Work out the finished part from the listing and answer in its coordinate system (mm). Face numbers are marked on the shaded views. A direction names the side the tool comes from. Coordinates: 2 decimals unless noted, no trailing zeros. Order: outer loops, then holes, each group sorted by start corner. A loop starts at its lowest first (then second) coordinate and runs counter-clockwise, first axis right, second up. Notation, with made-up numbers: (63, 68) -> (95, 68) arc R9 cw to (95, 76) -> close; hole circle Ø3 at (-15.5, 88.25). An arc over 180 degrees is marked (long way). Answer as CSV lines item,"result". Start each with the question number.
Item 1: Section A-A (y = 56.5) is taken. Count the separate pieces of the cut face and the enclosed holes in it, then the cut area to 3 significant figures.
Item 2: For a pull along X with two mould halves and no side action, classify the marked faces 1, 2, 3 and 4 as pulls with the +X half, pulls with the -X half, needs draft (parallel to the pull), parting line crosses it, or undercut.
Item 3: Straight lines are drawn through the part: L1, parallel to X at y = 56.75, z = 54; L2, parallel to Z at x = 24, y = 56.75; L3, parallel to Y at x = -36.5, z = 60. For each, find the intervals that lie inside material, in ascending order.
Item 4: Which of the six approach directions +Z, -Z, +X, -X, +Y, -Y give full straight-line access (tool end or side, diameter ignored) to the marked faces 5, 6, 7, 8 and 9?
Item 5: Section D-D (x = 26) is taken. Write down the section's boundary in (y, z).
Item 6: Each of these flat-tipped pins is pushed along its axis until it touches: pin 1 Ø5 at (x, z) = (19, 73) entering from +Y; pin 2 Ø0.7 at (x, y) = (3, 60.5) entering from +Z; pin 3 Ø1.8 at (y, z) = (60, 58) entering from -X. Where does it stop, or does it pass through?
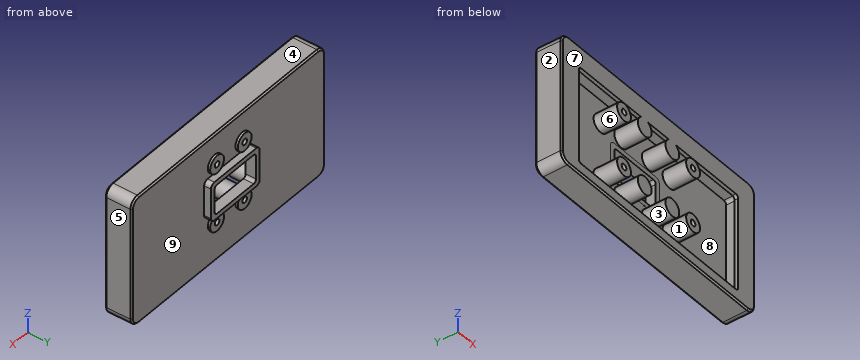
```python
from build123d import *

# Parameters (mm, degrees)
BOSS_EXTRUDE1_START  = 50
BOSS_EXTRUDE1_DEPTH  = 9.2
CHAMFER1_SIZE        = 0.5
CHAMFER2_SIZE        = 0.5
BOSS_EXTRUDE2_START  = 49
BOSS_EXTRUDE2_DEPTH  = 9
BOSS_EXTRUDE3_START  = 50
SKETCH3_R            = 3
BOSS_EXTRUDE3_DEPTH  = 8.01
BOSS_EXTRUDE4_START  = 49
SKETCH4_R            = 1
BOSS_EXTRUDE4_DEPTH  = 9.4
BOSS_EXTRUDE5_START  = 50
SKETCH5_R            = 3
BOSS_EXTRUDE5_DEPTH  = 8.01
BOSS_EXTRUDE6_START  = 49
SKETCH6_R            = 1
BOSS_EXTRUDE6_DEPTH  = 9.4
BOSS_EXTRUDE7_START  = 50
SKETCH7_R            = 3
BOSS_EXTRUDE7_DEPTH  = 8.01
BOSS_EXTRUDE8_START  = 49
SKETCH8_R            = 1
BOSS_EXTRUDE8_DEPTH  = 9.4
BOSS_EXTRUDE9_START  = 50
SKETCH9_R            = 3
BOSS_EXTRUDE9_DEPTH  = 8.01
BOSS_EXTRUDE10_START = 49
SKETCH10_R           = 1
BOSS_EXTRUDE10_DEPTH = 9.4
BOSS_EXTRUDE11_START = 50
SKETCH11_R           = 3
BOSS_EXTRUDE11_DEPTH = 10
BOSS_EXTRUDE12_START = 51.5
SKETCH12_R           = 1
BOSS_EXTRUDE12_DEPTH = 9.5
BOSS_EXTRUDE13_START = 50
SKETCH13_R           = 3
BOSS_EXTRUDE13_DEPTH = 10
BOSS_EXTRUDE14_START = 51.5
SKETCH14_R           = 1
BOSS_EXTRUDE14_DEPTH = 9.5
BOSS_EXTRUDE15_START = 50
SKETCH15_R           = 3
BOSS_EXTRUDE15_DEPTH = 10
BOSS_EXTRUDE16_START = 51.5
SKETCH16_R           = 1
BOSS_EXTRUDE16_DEPTH = 9.5
BOSS_EXTRUDE17_START = 50
SKETCH17_R           = 3
BOSS_EXTRUDE17_DEPTH = 10
BOSS_EXTRUDE18_START = 51.5
SKETCH18_R           = 1
BOSS_EXTRUDE18_DEPTH = 9.5
BOSS_EXTRUDE19_START = 50
BOSS_EXTRUDE19_DEPTH = 1.2
BOSS_EXTRUDE20_START = 57.99
BOSS_EXTRUDE20_DEPTH = 3.51
BOSS_EXTRUDE21_START = 49
BOSS_EXTRUDE21_DEPTH = 13


with BuildPart() as part:
    # Sketch1 → Boss-Extrude1 (new body)
    with BuildSketch(Plane(origin=(0, 0, 0), x_dir=(1, 0, 0), z_dir=(0, 1, 0)).offset(BOSS_EXTRUDE1_START)):
        with BuildLine():
            Line((-39, -36), (39, -36))
            ThreePointArc((39, -36), (41.121320344, -36.878679656), (42, -39))
            Line((42, -39), (42, -77))
            ThreePointArc((42, -77), (41.121320344, -79.121320344), (39, -80))
            Line((39, -80), (-39, -80))
            ThreePointArc((-39, -80), (-41.121320344, -79.121320344), (-42, -77))
            Line((-42, -77), (-42, -39))
            ThreePointArc((-42, -39), (-41.121320344, -36.878679656), (-39, -36))
        make_face()
    extrude(amount=BOSS_EXTRUDE1_DEPTH)

    # Chamfer1
    chamfer1_edges = [part.edges().sort_by_distance(p)[0] for p in [
        (0, 50, 80),
        (-41.121320344, 50, 79.121320344),
        (-42, 50, 58),
        (-41.121320344, 50, 36.878679656),
        (0, 50, 36),
        (41.121320344, 50, 36.878679656),
        (42, 50, 58),
        (41.121320344, 50, 79.121320344),
    ]]
    chamfer(chamfer1_edges, length=CHAMFER1_SIZE)

    # Chamfer2
    chamfer2_edges = [part.edges().sort_by_distance(p)[0] for p in [
        (-41.121320344, 59.2, 79.121320344),
        (0, 59.2, 80),
        (41.121320344, 59.2, 79.121320344),
        (42, 59.2, 58),
        (41.121320344, 59.2, 36.878679656),
        (0, 59.2, 36),
        (-41.121320344, 59.2, 36.878679656),
        (-42, 59.2, 58),
    ]]
    chamfer(chamfer2_edges, length=CHAMFER2_SIZE)


with BuildPart() as body_2:
    # Sketch2 → Boss-Extrude2 (new body)
    with BuildSketch(Plane(origin=(0, 0, 0), x_dir=(1, 0, 0), z_dir=(0, 1, 0)).offset(BOSS_EXTRUDE2_START)):
        with BuildLine():
            Line((-38.6, -38.4), (38.6, -38.4))
            ThreePointArc((38.6, -38.4), (39.307106781, -38.692893219), (39.6, -39.4))
            Line((39.6, -39.4), (39.6, -76.6))
            ThreePointArc((39.6, -76.6), (39.307106781, -77.307106781), (38.6, -77.6))
            Line((38.6, -77.6), (-38.6, -77.6))
            ThreePointArc((-38.6, -77.6), (-39.307106781, -77.307106781), (-39.6, -76.6))
            Line((-39.6, -76.6), (-39.6, -39.4))
            ThreePointArc((-39.6, -39.4), (-39.307106781, -38.692893219), (-38.6, -38.4))
        make_face()
    extrude(amount=BOSS_EXTRUDE2_DEPTH)


with BuildPart() as part_1:
    add(part.part)

    # Combine1: cut body 2
    add(body_2.part, mode=Mode.SUBTRACT)

    # Sketch3 → Boss-Extrude3 (add)
    with BuildSketch(Plane(origin=(0, 0, 0), x_dir=(1, 0, 0), z_dir=(0, 1, 0)).offset(BOSS_EXTRUDE3_START)):
        with Locations(Location((-15, -50.5, 0), (0, 0, 90))):
            Circle(SKETCH3_R)
    extrude(amount=BOSS_EXTRUDE3_DEPTH)


with BuildPart() as body_2_2:
    # Sketch4 → Boss-Extrude4 (new body)
    with BuildSketch(Plane(origin=(0, 0, 0), x_dir=(1, 0, 0), z_dir=(0, 1, 0)).offset(BOSS_EXTRUDE4_START)):
        with Locations(Location((-15, -50.5, 0), (0, 0, 90))):
            Circle(SKETCH4_R)
    extrude(amount=BOSS_EXTRUDE4_DEPTH)


with BuildPart() as part_2:
    add(part_1.part)

    # Combine2: cut body 2 2
    add(body_2_2.part, mode=Mode.SUBTRACT)

    # Sketch5 → Boss-Extrude5 (add)
    with BuildSketch(Plane(origin=(0, 0, 0), x_dir=(1, 0, 0), z_dir=(0, 1, 0)).offset(BOSS_EXTRUDE5_START)):
        with Locations(Location((-15, -69.5, 0), (0, 0, 90))):
            Circle(SKETCH5_R)
    extrude(amount=BOSS_EXTRUDE5_DEPTH)


with BuildPart() as body_2_3:
    # Sketch6 → Boss-Extrude6 (new body)
    with BuildSketch(Plane(origin=(0, 0, 0), x_dir=(1, 0, 0), z_dir=(0, 1, 0)).offset(BOSS_EXTRUDE6_START)):
        with Locations(Location((-15, -69.5, 0), (0, 0, 90))):
            Circle(SKETCH6_R)
    extrude(amount=BOSS_EXTRUDE6_DEPTH)


with BuildPart() as part_3:
    add(part_2.part)

    # Combine3: cut body 2 3
    add(body_2_3.part, mode=Mode.SUBTRACT)

    # Sketch7 → Boss-Extrude7 (add)
    with BuildSketch(Plane(origin=(0, 0, 0), x_dir=(1, 0, 0), z_dir=(0, 1, 0)).offset(BOSS_EXTRUDE7_START)):
        with Locations(Location((15, -50.5, 0), (0, 0, 90))):
            Circle(SKETCH7_R)
    extrude(amount=BOSS_EXTRUDE7_DEPTH)


with BuildPart() as body_2_4:
    # Sketch8 → Boss-Extrude8 (new body)
    with BuildSketch(Plane(origin=(0, 0, 0), x_dir=(1, 0, 0), z_dir=(0, 1, 0)).offset(BOSS_EXTRUDE8_START)):
        with Locations(Location((15, -50.5, 0), (0, 0, 90))):
            Circle(SKETCH8_R)
    extrude(amount=BOSS_EXTRUDE8_DEPTH)


with BuildPart() as part_4:
    add(part_3.part)

    # Combine4: cut body 2 4
    add(body_2_4.part, mode=Mode.SUBTRACT)

    # Sketch9 → Boss-Extrude9 (add)
    with BuildSketch(Plane(origin=(0, 0, 0), x_dir=(1, 0, 0), z_dir=(0, 1, 0)).offset(BOSS_EXTRUDE9_START)):
        with Locations(Location((15, -69.5, 0), (0, 0, 90))):
            Circle(SKETCH9_R)
    extrude(amount=BOSS_EXTRUDE9_DEPTH)


with BuildPart() as body_2_5:
    # Sketch10 → Boss-Extrude10 (new body)
    with BuildSketch(Plane(origin=(0, 0, 0), x_dir=(1, 0, 0), z_dir=(0, 1, 0)).offset(BOSS_EXTRUDE10_START)):
        with Locations(Location((15, -69.5, 0), (0, 0, 90))):
            Circle(SKETCH10_R)
    extrude(amount=BOSS_EXTRUDE10_DEPTH)


with BuildPart() as part_5:
    add(part_4.part)

    # Combine5: cut body 2 5
    add(body_2_5.part, mode=Mode.SUBTRACT)

    # Sketch11 → Boss-Extrude11 (add)
    with BuildSketch(Plane(origin=(0, 0, 0), x_dir=(1, 0, 0), z_dir=(0, 1, 0)).offset(BOSS_EXTRUDE11_START)):
        with Locations(Location((-6, -50, 0), (0, 0, 90))):
            Circle(SKETCH11_R)
    extrude(amount=BOSS_EXTRUDE11_DEPTH)


with BuildPart() as body_2_6:
    # Sketch12 → Boss-Extrude12 (new body)
    with BuildSketch(Plane(origin=(0, 0, 0), x_dir=(1, 0, 0), z_dir=(0, 1, 0)).offset(BOSS_EXTRUDE12_START)):
        with Locations(Location((-6, -50, 0), (0, 0, 270))):
            Circle(SKETCH12_R)
    extrude(amount=BOSS_EXTRUDE12_DEPTH)


with BuildPart() as part_6:
    add(part_5.part)

    # Combine6: cut body 2 6
    add(body_2_6.part, mode=Mode.SUBTRACT)

    # Sketch13 → Boss-Extrude13 (add)
    with BuildSketch(Plane(origin=(0, 0, 0), x_dir=(1, 0, 0), z_dir=(0, 1, 0)).offset(BOSS_EXTRUDE13_START)):
        with Locations(Location((-6, -70, 0), (0, 0, 90))):
            Circle(SKETCH13_R)
    extrude(amount=BOSS_EXTRUDE13_DEPTH)


with BuildPart() as body_2_7:
    # Sketch14 → Boss-Extrude14 (new body)
    with BuildSketch(Plane(origin=(0, 0, 0), x_dir=(1, 0, 0), z_dir=(0, 1, 0)).offset(BOSS_EXTRUDE14_START)):
        with Locations(Location((-6, -70, 0), (0, 0, 270))):
            Circle(SKETCH14_R)
    extrude(amount=BOSS_EXTRUDE14_DEPTH)


with BuildPart() as part_7:
    add(part_6.part)

    # Combine7: cut body 2 7
    add(body_2_7.part, mode=Mode.SUBTRACT)

    # Sketch15 → Boss-Extrude15 (add)
    with BuildSketch(Plane(origin=(0, 0, 0), x_dir=(1, 0, 0), z_dir=(0, 1, 0)).offset(BOSS_EXTRUDE15_START)):
        with Locations(Location((6, -50, 0), (0, 0, 90))):
            Circle(SKETCH15_R)
    extrude(amount=BOSS_EXTRUDE15_DEPTH)


with BuildPart() as body_2_8:
    # Sketch16 → Boss-Extrude16 (new body)
    with BuildSketch(Plane(origin=(0, 0, 0), x_dir=(1, 0, 0), z_dir=(0, 1, 0)).offset(BOSS_EXTRUDE16_START)):
        with Locations(Location((6, -50, 0), (0, 0, 270))):
            Circle(SKETCH16_R)
    extrude(amount=BOSS_EXTRUDE16_DEPTH)


with BuildPart() as part_8:
    add(part_7.part)

    # Combine8: cut body 2 8
    add(body_2_8.part, mode=Mode.SUBTRACT)

    # Sketch17 → Boss-Extrude17 (add)
    with BuildSketch(Plane(origin=(0, 0, 0), x_dir=(1, 0, 0), z_dir=(0, 1, 0)).offset(BOSS_EXTRUDE17_START)):
        with Locations(Location((6, -70, 0), (0, 0, 90))):
            Circle(SKETCH17_R)
    extrude(amount=BOSS_EXTRUDE17_DEPTH)


with BuildPart() as body_2_9:
    # Sketch18 → Boss-Extrude18 (new body)
    with BuildSketch(Plane(origin=(0, 0, 0), x_dir=(1, 0, 0), z_dir=(0, 1, 0)).offset(BOSS_EXTRUDE18_START)):
        with Locations(Location((6, -70, 0), (0, 0, 270))):
            Circle(SKETCH18_R)
    extrude(amount=BOSS_EXTRUDE18_DEPTH)


with BuildPart() as part_9:
    add(part_8.part)

    # Combine9: cut body 2 9
    add(body_2_9.part, mode=Mode.SUBTRACT)

    # Sketch19 → Boss-Extrude19 (add)
    with BuildSketch(Plane(origin=(0, 0, 0), x_dir=(1, 0, 0), z_dir=(0, 1, 0)).offset(BOSS_EXTRUDE19_START)):
        with BuildLine():
            Line((-38.59, -38.39), (38.59, -38.39))
            ThreePointArc((38.59, -38.39), (39.297106781, -38.682893219), (39.59, -39.39))
            Line((39.59, -39.39), (39.59, -76.61))
            ThreePointArc((39.59, -76.61), (39.297106781, -77.317106781), (38.59, -77.61))
            Line((38.59, -77.61), (-38.59, -77.61))
            ThreePointArc((-38.59, -77.61), (-39.297106781, -77.317106781), (-39.59, -76.61))
            Line((-39.59, -76.61), (-39.59, -39.39))
            ThreePointArc((-39.59, -39.39), (-39.297106781, -38.682893219), (-38.59, -38.39))
        make_face()
        with BuildLine():
            Line((-33.6, -39.6), (33.6, -39.6))
            ThreePointArc((33.6, -39.6), (34.307106781, -39.892893219), (34.6, -40.6))
            Line((34.6, -40.6), (34.6, -71.6))
            ThreePointArc((34.6, -71.6), (34.307106781, -72.307106781), (33.6, -72.6))
            Line((33.6, -72.6), (-33.6, -72.6))
            ThreePointArc((-33.6, -72.6), (-34.307106781, -72.307106781), (-34.6, -71.6))
            Line((-34.6, -71.6), (-34.6, -40.6))
            ThreePointArc((-34.6, -40.6), (-34.307106781, -39.892893219), (-33.6, -39.6))
        make_face(mode=Mode.SUBTRACT)
    extrude(amount=BOSS_EXTRUDE19_DEPTH)

    # Sketch20 → Boss-Extrude20 (add)
    with BuildSketch(Plane(origin=(0, 0, 0), x_dir=(1, 0, 0), z_dir=(0, 1, 0)).offset(BOSS_EXTRUDE20_START)):
        with BuildLine():
            Line((-9.1, -53.4), (9.1, -53.4))
            ThreePointArc((9.1, -53.4), (10.160660172, -53.839339828), (10.6, -54.9))
            Line((10.6, -54.9), (10.6, -65.1))
            ThreePointArc((10.6, -65.1), (10.160660172, -66.160660172), (9.1, -66.6))
            Line((9.1, -66.6), (-9.1, -66.6))
            ThreePointArc((-9.1, -66.6), (-10.160660172, -66.160660172), (-10.6, -65.1))
            Line((-10.6, -65.1), (-10.6, -54.9))
            ThreePointArc((-10.6, -54.9), (-10.160660172, -53.839339828), (-9.1, -53.4))
        make_face()
    extrude(amount=BOSS_EXTRUDE20_DEPTH)


with BuildPart() as body_2_10:
    # Sketch21 → Boss-Extrude21 (new body)
    with BuildSketch(Plane(origin=(0, 0, 0), x_dir=(1, 0, 0), z_dir=(0, 1, 0)).offset(BOSS_EXTRUDE21_START)):
        with BuildLine():
            Line((-8, -55), (8, -55))
            ThreePointArc((8, -55), (8.707106781, -55.292893219), (9, -56))
            Line((9, -56), (9, -64))
            ThreePointArc((9, -64), (8.707106781, -64.707106781), (8, -65))
            Line((8, -65), (-8, -65))
            ThreePointArc((-8, -65), (-8.707106781, -64.707106781), (-9, -64))
            Line((-9, -64), (-9, -56))
            ThreePointArc((-9, -56), (-8.707106781, -55.292893219), (-8, -55))
        make_face()
    extrude(amount=BOSS_EXTRUDE21_DEPTH)


with BuildPart() as part_10:
    add(part_9.part)

    # Combine10: cut body 2 10
    add(body_2_10.part, mode=Mode.SUBTRACT)


solid = part_10.part
```
Checked values:
1,separate pieces,"9"
1,enclosed holes,"9"
1,area,"786 mm^2"
2,face 1,"undercut"
2,face 2,"pulls with the -X half"
2,face 3,"undercut"
2,face 4,"needs draft"
3,L1,"x = -42 to -39.6, 39.6 to 42"
3,L2,"z = 36 to 38.4, 77.6 to 80"
3,L3,"y = 50 to 51.2, 58 to 59.2"
4,face 5,"+Z, -Z, +X, +Y, -Y"
4,face 6,"-Y"
4,face 7,"+Z, -Z, +X, -X, -Y"
4,face 8,"none"
4,face 9,"+Y"
5,outline,"(50, 36.5) -> (50.5, 36) -> (58.7, 36) -> (59.2, 36.5) -> (59.2, 79.5) -> (58.7, 80) -> (50.5, 80) -> (50, 79.5) -> (50, 72.6) -> (51.2, 72.6) -> (51.2, 77.6) -> (58, 77.6) -> (58, 38.4) -> (51.2, 38.4) -> (51.2, 39.6) -> (50, 39.6) -> close"
6,pin 1,"stops at y = 59.2"
6,pin 2,"stops at z = 66.6"
6,pin 3,"stops at x = -41.6"
